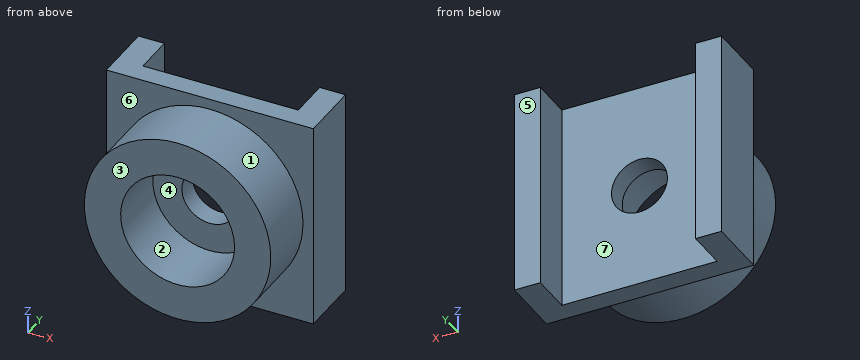
```python
from build123d import *

# Parameters (mm, degrees)
ESQUISSE1_R        = 4.5
ESQUISSE1_R_2      = 2.75
BOSS_EXTRU_1_DEPTH = 3
ESQUISSE3_W        = 10
ESQUISSE3_H        = 10
ESQUISSE3_R        = 1.35
BOSS_EXTRU_2_DEPTH = 1
ESQUISSE4_W        = 1.25
ESQUISSE4_H        = 10
BOSS_EXTRU_3_DEPTH = 2


with BuildPart() as part:
    # Esquisse1 → Boss.-Extru.1 (new body)
    with BuildSketch(Plane(origin=(0, 0, 0), x_dir=(1, 0, 0), z_dir=(0, 1, 0))):
        with Locations(Location((0, 0, 0), (0, 0, 270))):
            Circle(ESQUISSE1_R)
        with Locations(Location((0, 0, 0), (0, 0, 270))):
            Circle(ESQUISSE1_R_2, mode=Mode.SUBTRACT)
    extrude(amount=-BOSS_EXTRU_1_DEPTH)

    # Esquisse3 → Boss.-Extru.2 (add)
    with BuildSketch(Plane(origin=(0, 0, 0), x_dir=(1, 0, 0), z_dir=(0, 1, 0))):
        Rectangle(ESQUISSE3_W, ESQUISSE3_H)
        with Locations(Location((0, 0, 0), (0, 0, 270))):
            Circle(ESQUISSE3_R, mode=Mode.SUBTRACT)
    extrude(amount=BOSS_EXTRU_2_DEPTH)

    # Esquisse4 → Boss.-Extru.3 (add)
    with BuildSketch(Plane(origin=(0, 1, 0), x_dir=(1, 0, 0), z_dir=(0, 1, 0))):
        with Locations((-4.375, 0)):
            Rectangle(ESQUISSE4_W, ESQUISSE4_H)
        with Locations((4.375, 0)):
            Rectangle(ESQUISSE4_W, ESQUISSE4_H)
    extrude(amount=BOSS_EXTRU_3_DEPTH)


solid = part.part
```
For this review, take the finished solid that the model builds, in its own axes (mm). Face numbers are marked on the shaded views. A direction names the side the tool comes from. Coordinates: 2 decimals unless noted, no trailing zeros. Write each loop counter-clockwise with the first axis right and the second up, starting at its lowest first coordinate (ties: lowest second). Pieces come first, ordered by that corner, then holes.
(1) Add section A-A on y = 1.2. Give the boundary of the cut face in (x, z).
(2) Add section B-B on x = 0. Give the boundary of the cut face in (y, z).
(3) The part is to be moulded in two halves that separate along Z. For the marked faces 1, 2, 3 and 4, say which applies: +Z half, -Z half, draft (parallel to the pull), parting line (faces both ways), or undercut.
(4) Add section D-D on y = -1.45. Give the boundary of the cut face in (x, z), then the cut area to 3 significant figures.
(5) Tool access review of the marked faces 5, 6 and 7: name each direction out of +Z, -Z, +X, -X, +Y, -Y from which nothing blocks a thin tool from reaching the whole face with its end or side.
(6) Wall thickness on probe 1 along X at (y, z) = (0.85, 0); probe 2 along Y at (x, z) = (-0.75, -2); probe 3 along Y at (x, z) = (0.5, -2.75): over which ranges is each line inside the solid? List them lowest first.
(7) Add section C-C on z = 0. Give the boundary of the cut face in (x, y), then the cut area to 3 significant figures.
(8) For pin 1 Ø2 at (x, z) = (2.5, -4) entering from +Y; pin 2 Ø2 at (x, y) = (-2, 1.5) entering from -Z; pin 3 Ø5 at (x, z) = (0, 0) entering from -Y; pin 4 Ø2 at (y, z) = (-1.5, -4) entering from +X, all flat-tipped, find the tip position at first contact; note any pin that passes through.
Answer sheet:
1. outline: (-5, -5) - (-3.75, -5) - (-3.75, 5) - (-5, 5) - close; (3.75, -5) - (5, -5) - (5, 5) - (3.75, 5) - close
2. outline: (-3, -4.5) - (0, -4.5) - (0, -5) - (1, -5) - (1, -1.35) - (0, -1.35) - (0, -2.75) - (-3, -2.75) - close; (-3, 2.75) - (0, 2.75) - (0, 1.35) - (1, 1.35) - (1, 5) - (0, 5) - (0, 4.5) - (-3, 4.5) - close
3. face 1: parting line
3. face 2: undercut
3. face 3: draft
3. face 4: undercut
4. outline: circle Ø9 at (0, 0); hole circle Ø5.5 at (0, 0)
4. area: 39.9 mm2
5. face 5: +Z, -Z, +X, -X, +Y
5. face 6: -Y
5. face 7: +Z, -Z, +Y
6. probe 1: x = -5 to -1.35, 1.35 to 5
6. probe 2: y = 0 to 1
6. probe 3: y = -3 to 1
7. outline: (-5, 0) - (-4.5, 0) - (-4.5, -3) - (-2.75, -3) - (-2.75, 0) - (-1.35, 0) - (-1.35, 1) - (-3.75, 1) - (-3.75, 3) - (-5, 3) - close; (1.35, 0) - (2.75, 0) - (2.75, -3) - (4.5, -3) - (4.5, 0) - (5, 0) - (5, 3) - (3.75, 3) - (3.75, 1) - (1.35, 1) - close
7. area: 22.8 mm2
8. pin 1: stops at y = 1
8. pin 2: stops at z = -5
8. pin 3: stops at y = 0
8. pin 4: stops at x = 3.35
